Input: part model. Units: mm. Frame: model coordinates. A direction names the side the tool comes from. Give positions to 0.01 mm unless a question says otherwise; leave off trailing zeros. Loops run counter-clockwise (first coordinate to the right, second up) from the corner with the lowest first, then second, coordinate; pieces in that order, holes last. Notation, with made-up numbers: M -15.75,-4.5 L -2.75,-4.5 A19 ccw -2.75,1.5 Z; hole C 24.25,70 d8. An arc over 180 degrees is marked long. Answer as a JSON object with one key per item and string values. Group by question number.
1) Section query C-C on z = 3.75. Return loops of the section in (x, y), plus the area to 3 significant figures.
2) Access query for faces 1 (the flat face through (1.2, -1.2, 0)), 2 (the flat face through (-1.2, 1.2, 1)), 3 (the cylindrical face through (-6, 0, 2)). Directions: +Z, -Z, +X, -X, +Y, -Y. A direction counts if a zero-diameter tool reaches every point of the face in a straight line with its end or side. Return the directions, or none.
3) Draft query along Y for faces 4 (the cylindrical face through (-1.5, 0.07, 0.51)), 5 (the cylindrical face through (6.466, -2.681, 5.507)), 6 (the flat face through (6, 2, 5)). Return one class per face: +Y half, -Y half, draft (parallel to the pull), parting line (faces both ways), or undercut.
4) Section query A-A on y = 0. Return loops of the section in (x, z).
5) Section query D-D on x = -2.5. Return loops of the section in (y, z).
6) First-contact query: P1, Ø3, axis at x = -4.5, z = 1.5, coming from the +Y side; P2, Ø3, axis at x = -5, z = 3, coming from the +Y side; P3, Ø3, axis at y = 4.5, z = 5.5, coming from the -X side; P4, Ø1.8, axis at x = 0, y = 0, coming from the -Z side. Flat tips, straight axial feed; report the tip coordinate or a pass-through.
7) Ray query, L1, parallel to Y at x = 0, z = 2.3; L2, parallel to Z at x = 3.25, y = -5.5; L3, parallel to Z at x = 3.25, y = -0.25. Return the intervals inside material, ascending.
from build123d import *

# Parameters (mm, degrees)
SKETCH_1_R          = 6
EXTRUDE_1_DEPTH     = 1
SKETCH_2_R          = 6
SKETCH_2_R_2        = 4.95
EXTRUDE_2_DEPTH     = 5
SKETCH_3_R          = 7
EXTRUDE_3_DEPTH     = 1
CUT_EXTRUDE_START   = -5
SKETCH_5_R          = 4.95
CUT_EXTRUDE_1_DEPTH = 5
SKETCH_6_R          = 1.5
CUT_EXTRUDE_2_DEPTH = 1


with BuildPart() as part:
    # Эскиз1 → Бобышка-Вытянуть1 (new body)
    with BuildSketch(Plane.XY):
        Circle(SKETCH_1_R)
    extrude(amount=EXTRUDE_1_DEPTH)

    # Эскиз2 → Бобышка-Вытянуть2 (add)
    with BuildSketch(Plane.XY.offset(1)):
        Circle(SKETCH_2_R)
        Circle(SKETCH_2_R_2, mode=Mode.SUBTRACT)
    extrude(amount=EXTRUDE_2_DEPTH)

    # Эскиз3 → Бобышка-Вытянуть3 (add)
    with BuildSketch(Plane.XY.offset(6)):
        Circle(SKETCH_3_R)
    extrude(amount=-EXTRUDE_3_DEPTH)

    # Эскиз5 → Вырез-Вытянуть1 (cut)
    with BuildSketch(Plane.XY.offset(6).offset(CUT_EXTRUDE_START)):
        Circle(SKETCH_5_R)
    extrude(amount=CUT_EXTRUDE_1_DEPTH, mode=Mode.SUBTRACT)

    # Эскиз6 → Вырез-Вытянуть2 (cut)
    with BuildSketch(Plane.XY.offset(1)):
        Circle(SKETCH_6_R)
    extrude(amount=-CUT_EXTRUDE_2_DEPTH, mode=Mode.SUBTRACT)


solid = part.part
Output:
{
 "1": {"outline": "C 0,0 d12; hole C 0,0 d9.9", "area": "36.1 mm^2"},
 "2": {"face 1": "-Z, +X, -X, +Y, -Y", "face 2": "+Z", "face 3": "-Z"},
 "3": {"face 4": "undercut", "face 5": "parting line", "face 6": "draft"},
 "4": {"outline": "M -7,5 L -6,5 L -6,0 L -1.5,0 L -1.5,1 L -4.95,1 L -4.95,6 L -7,6 Z; M 1.5,0 L 6,0 L 6,5 L 7,5 L 7,6 L 4.95,6 L 4.95,1 L 1.5,1 Z"},
 "5": {"outline": "M -6.54,5 L -5.45,5 L -5.45,0 L 5.45,0 L 5.45,5 L 6.54,5 L 6.54,6 L 4.27,6 L 4.27,1 L -4.27,1 L -4.27,6 L -6.54,6 Z"},
 "6": {"P1": "stops at y = 5.2", "P2": "stops at y = 4.87", "P3": "stops at x = -6.32", "P4": "passes through"},
 "7": {"L1": "y = -6 to -4.95, 4.95 to 6", "L2": "z = 5 to 6", "L3": "z = 0 to 1"}
}
